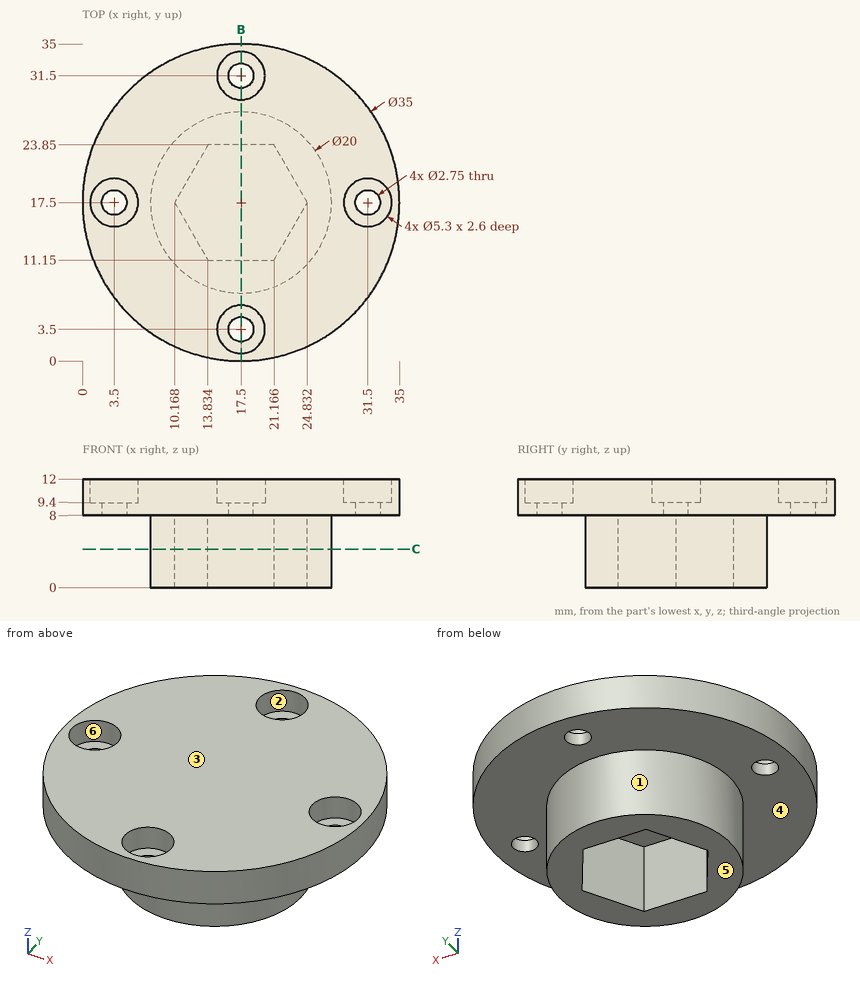
For this review, use the dimensioned drawing (mm, ordinates from the lowest corner) and the shaded views. A direction names the side the tool comes from. Round coordinates to 2 decimals unless told otherwise and drop trailing zeros. Write each loop counter-clockwise with the first axis right and the second up, starting at its lowest first coordinate (ties: lowest second). Pieces come first, ordered by that corner, then holes. Notation, with made-up numbers: (44.5, -32.5) - (98.5, -32.5) arc R24 ccw to (98.5, 6.5) - close; hole circle Ø4 at (69, 23). An arc over 180 degrees is marked (long way). Use CSV: the item, a comma, the result in double quotes.
1) For the marked faces 4, 5 and 6, list the 3-axis set-ups (+Z, -Z, +X, -X, +Y, -Y) from which the entire face can be reached by the end or side of a thin tool; tool diameter is ignored.
Conclusion:
face 4,"-Z"
face 5,"-Z, +X, -X, +Y, -Y"
face 6,"+Z"
2) Add section B-B on x = 17.5. Count the separate pieces of the cut face and the enclosed holes in it, and give its area (3 significant figures).
Conclusion:
separate pieces,"3"
enclosed holes,"0"
area,"163 mm^2"
3) Add section C-C on z = 4.25. Write out the cut boundary in (x, y).
Conclusion:
outline,"circle Ø20 at (17.5, 17.5); hole (10.17, 17.5) - (13.83, 11.15) - (21.17, 11.15) - (24.83, 17.5) - (21.17, 23.85) - (13.83, 23.85) - close"
4) The part is to be moulded in two halves that separate along Y. For the marked faces 1, 2 and 3, say which applies: pulls with the +Y half, pulls with the -Y half, needs draft (parallel to the pull), parting line crosses it, or undercut.
Conclusion:
face 1,"parting line crosses it"
face 2,"undercut"
face 3,"needs draft"
5) Wall thickness on line 1 along Y through (x, z) = (17.5, 11.1); line 2 along Y through (x, z) = (17.5, 8.4) (1 decimal); line 3 along Z through (x, y) = (14, 17): over which ranges is each line inside the solid? List them lowest first. Write a range as from..to.
Conclusion:
line 1,"y = 0..0.85, 6.15..28.85, 34.15..35"
line 2,"y = 0..2.1, 4.9..30.1, 32.9..35"
line 3,"z = 8..12"
6) Clearance check with flat-ended pins moving along their axes: pin 1 Ø3.5 at (x, z) = (19, 2) entering from -Y; pin 2 Ø5 at (x, y) = (31.5, 17.5) entering from +Z; pin 3 Ø3 at (x, y) = (17.5, 31.5) entering from -Z. State where each tip first meets the part, or that it passes through.
Conclusion:
pin 1,"stops at y = 7.5"
pin 2,"stops at z = 9.4"
pin 3,"stops at z = 8"
